Read the model definition and answer for the solid it produces. Units are mm, in the model's axes. A direction names the side the tool comes from. Coordinates: 2 decimals unless noted, no trailing zeros. Order: outer loops, then holes, each group sorted by start corner. A loop starts at its lowest first (then second) coordinate and runs counter-clockwise, first axis right, second up. Notation, with made-up numbers: M 70,42 L 99,42 A21 cw 99,68 Z; hole C -5,72.5 d4. An arc over 180 degrees is marked long. Put each result on its own line as item: value.
Autodesk Inventor part; units mm, degrees
ref_plane "YZ Plane" through (0, 0, 0) normal (1, 0, 0) x (0, 1, 0)
ref_plane "XZ Plane" through (0, 0, 0) normal (0, 1, 0) x (-1, 0, 0)
ref_plane "XY Plane" through (0, 0, 0) normal (0, 0, 1) x (1, 0, 0)
sketch "スケッチ1" plane through (0, 0, 0) normal (0, 0, 1) x (1, 0, 0)
  circle A0 centre (0, 0) radius 1.5
  dimension "d0" = 3
extrude "押し出し1" add sketch "スケッチ1" along normal blind 6
sketch "スケッチ2" plane through (0, 0, 6) normal (0, 0, 1) x (1, 0, 0)
  circle A0 centre (0, 0) radius 1.5
  circle A1 centre (0, 0) radius 3
  dimension "d3" = 6
extrude "押し出し2" add sketch "スケッチ2" along normal blind 2 contours A0 | A1
fillet "フィレット1" radius 2 1 edges at (-3, 0, 8)
thread "ねじ1"
sketch "スケッチ3" plane through (0, 0, 0) normal (0, 0, -1) x (-1, 0, 0)
  circle A0 centre (0, 0) radius 1.5
extrude "押し出し3" add sketch "スケッチ3" along normal blind 9
sketch "スケッチ4" plane through (0, 0, -9) normal (0, 0, -1) x (-1, 0, 0)
  circle A0 centre (0, 0) radius 1.5
extrude "押し出し4" add sketch "スケッチ4" along normal blind 5
sketch "スケッチ5" plane through (0, 0, 8) normal (0, 0, 1) x (1, 0, 0)
  line L0 (0.8191, 1.1885) -> (1.4388, -0.1151)
  line L1 (1.4388, -0.1151) -> (0.6197, -1.3036)
  line L2 (0.6197, -1.3036) -> (-0.8191, -1.1885)
  line L3 (-0.8191, -1.1885) -> (-1.4388, 0.1151)
  line L4 (-1.4388, 0.1151) -> (-0.6197, 1.3036)
  line L5 (-0.6197, 1.3036) -> (0.8191, 1.1885)
  point P0 (0, 0)
  point P1 (0, 0)
  dimension "d13" = 2.5
extrude "押し出し5" cut sketch "スケッチ5" against normal blind 1.3
properties part number "SB　20mmなべネジ" material "Steel, Mild"
Q1. For a pull along X with two mould halves and no side action, classify faces 1 (the face through (-1.125, -0.546, 7.351)), 2 (the face through (1.3, -1.3, 6)) as +X half, -X half, draft (parallel to the pull), parting line (faces both ways), or undercut.
Answers below:
face 1: undercut
face 2: draft
Q2. Given pin 1 (1.3 mm diameter, centred on x = 0.5, y = 0, fed in from +Z); pin 2 (3 mm diameter, centred on x = -0.5, y = 1.5, fed in from -Z); pin 3 (2 mm diameter, centred on x = -1.5, z = 6, fed in from -Y), each flat-ended and moving along its own axis, determine where each tip first touches the part or whether it passes through.
Answers below:
pin 1: stops at z = 6.7
pin 2: stops at z = -14
pin 3: stops at y = -2.96
Q3. A tool of negligible diameter and unlimited length cuts with its end or side. For faces 3 (the face through (-0.09, -1.247, 7.351)), 4 (the face through (0, 0, -14)), from which of +Z, -Z, +X, -X, +Y, -Y can it reach the whole face along a straight path? Write none if from no direction.
Answers below:
face 3: +Z
face 4: -Z, +X, -X, +Y, -Y
Q4. Find section A-A on z = -5. Write down the section's boundary in (x, y), plus the area to 3 significant figures.
Answers below:
outline: C 0,0 d3
area: 7.07 mm^2
Q5. Consider line 1 along Z through (x, y) = (0.5, 1); line 2 along Y through (x, z) = (0, -9). Determine where each line is inside the solid, lowest interval first.
Answers below:
line 1: z = -14 to 6.7
line 2: y = -1.5 to 1.5
